Can you work these out from the model? Positions are in its coordinate system, mm. Give positions to 0.01 mm unless a question says otherwise; leave off trailing zeros. Write each loop counter-clockwise with the first axis right and the second up, starting at its lowest first coordinate (ties: lowest second). Pieces come first, ordered by that corner, then holes. Notation, with made-up numbers: (81, -23) -> (106, -23) arc R6 ccw to (106, -19) -> close; hole circle Ø2 at (-36.5, 48.5). An arc over 180 degrees is marked (long way). Answer as CSV lines item,"result". Start each with the question number.
1. If we section it at B-B on x = 0.5: Write out the boundary of the cut face in (y, z), plus the area to 3 significant figures.
2. I need wall thicknesses on line 1 (Y direction, x = -2.5, z = 1.4); line 2 (X direction, y = -0.5, z = 0.3); line 3 (Y direction, x = 4, z = 1.45). Which ranges of each line are inside material? Lowest first, please. Write a range as [from, to].
3. If we section it at A-A on y = -1.25: Write out the boundary of the cut face in (x, z), plus the area to 3 significant figures.
4. If we section it at D-D on z = 1.3: Count the separate pieces of the cut face and the enclosed holes in it, plus the area to 3 significant figures.
5. If we section it at C-C on y = 4.5: Write out the boundary of the cut face in (x, z), plus the area to 3 significant figures.
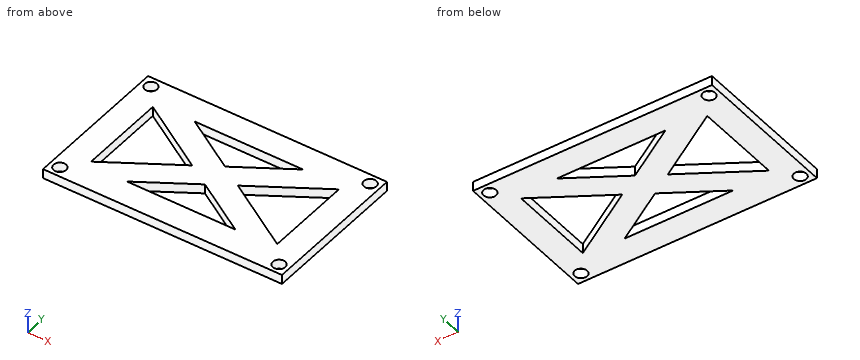
```python
from build123d import *

# Parameters (mm, degrees)
SKETCH2_W           = 40.2336
SKETCH2_H           = 25.019
SKETCH2_R           = 1.05
BOSS_EXTRUDE1_DEPTH = 1.5875


with BuildPart() as part:
    # Sketch2 → Boss-Extrude1 (new body)
    with BuildSketch(Plane.XY):
        Rectangle(SKETCH2_W, SKETCH2_H)
        with Locations((-18.4568, 10.8495)):
            Circle(SKETCH2_R, mode=Mode.SUBTRACT)
        with Locations(Location((-18.4568, -10.8495, 0), (0, 0, 180))):
            Circle(SKETCH2_R, mode=Mode.SUBTRACT)
        with Locations((18.4568, -10.8495)):
            Circle(SKETCH2_R, mode=Mode.SUBTRACT)
        with Locations(Location((18.4568, 10.8495, 0), (0, 0, 180))):
            Circle(SKETCH2_R, mode=Mode.SUBTRACT)
        Polygon((15.6718, -7.352568033), (3.847974859, 0), (15.6718, 7.352568033), align=None, mode=Mode.SUBTRACT)
        Polygon((9.120723619, -8.0645), (0, -2.392837901), (-9.120723619, -8.0645), align=None, mode=Mode.SUBTRACT)
        Polygon((9.120723619, 8.0645), (-9.120723619, 8.0645), (0, 2.392837901), align=None, mode=Mode.SUBTRACT)
        Polygon((-15.6718, 7.352568033), (-15.6718, -7.352568033), (-3.847974859, 0), align=None, mode=Mode.SUBTRACT)
    extrude(amount=BOSS_EXTRUDE1_DEPTH)


solid = part.part
```
Computed values:
1,outline,"(-12.51, 0) -> (-8.06, 0) -> (-8.06, 1.59) -> (-12.51, 1.59) -> close; (-2.7, 0) -> (2.7, 0) -> (2.7, 1.59) -> (-2.7, 1.59) -> close; (8.06, 0) -> (12.51, 0) -> (12.51, 1.59) -> (8.06, 1.59) -> close"
1,area,"22.7 mm2"
2,line 1,"y = [-12.51, -8.06], [-3.95, 3.95], [8.06, 12.51]"
2,line 2,"x = [-20.12, -15.67], [-4.65, 4.65], [15.67, 20.12]"
2,line 3,"y = [-12.51, -8.06], [-4.88, -0.09], [0.09, 4.88], [8.06, 12.51]"
3,outline,"(-20.12, 0) -> (-15.67, 0) -> (-15.67, 1.59) -> (-20.12, 1.59) -> close; (-5.86, 0) -> (5.86, 0) -> (5.86, 1.59) -> (-5.86, 1.59) -> close; (15.67, 0) -> (20.12, 0) -> (20.12, 1.59) -> (15.67, 1.59) -> close"
3,area,"32.7 mm2"
4,separate pieces,"1"
4,enclosed holes,"8"
4,area,"715 mm2"
5,outline,"(-20.12, 0) -> (-15.67, 0) -> (-15.67, 1.59) -> (-20.12, 1.59) -> close; (-11.08, 0) -> (-3.39, 0) -> (-3.39, 1.59) -> (-11.08, 1.59) -> close; (3.39, 0) -> (11.08, 0) -> (11.08, 1.59) -> (3.39, 1.59) -> close; (15.67, 0) -> (20.12, 0) -> (20.12, 1.59) -> (15.67, 1.59) -> close"
5,area,"38.5 mm2"
